Here's the drawing with two shaded views (mm, measured from the low corner). I have some questions. A direction names the side the tool comes from. Round coordinates to 2 decimals unless told otherwise and drop trailing zeros. Loops run counter-clockwise (first coordinate to the right, second up) from the corner with the lowest first, then second, coordinate; pieces in that order, holes last. Notation, with made-up numbers: M 7,37.5 L 65,37.5 A7 cw 65,46.5 Z; hole C 46.5,14 d9. An arc over 180 degrees is marked long. Write each question's results on one line, items separated by ' | '. Start each with the question number.
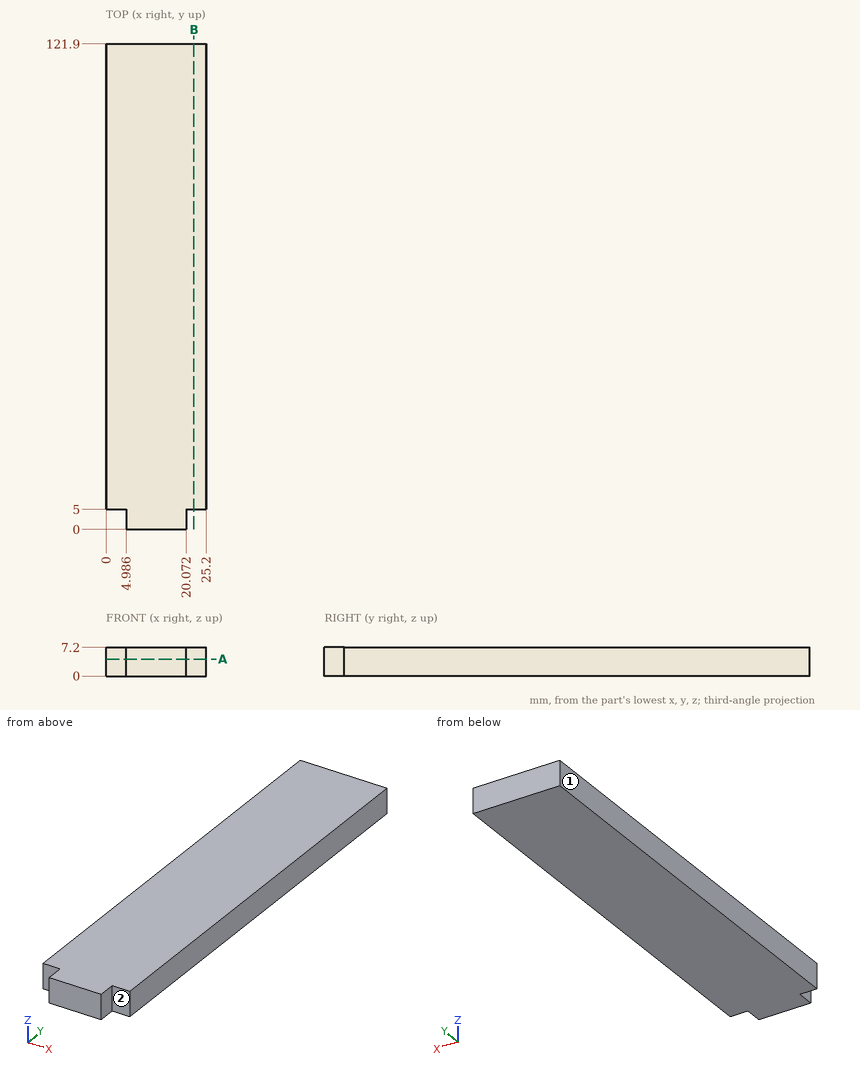
Item 1: Which directions (+Z, -Z, +X, -X, +Y, -Y) give clear straight access to the entire face, cutting with the end or side of a thin tool? Please do the marked faces 1 and 2.
Item 2: If we section it at A-A on z = 4.25: Please give me the cut outline in (x, y), and give its area (3 significant figures).
Item 3: I need wall thicknesses on L1, parallel to Y at x = 20.25, z = 5.75. Which ranges of the line are inside material? Lowest first, please.
Item 4: If we section it at B-B on x = 22: Please give me the cut outline in (y, z).
Item 5: I'm going to push flat-ended pins straight in: pin 1 (4 mm diameter, centred on x = 23, z = 4.5, fed in from -Y); pin 2 (1.5 mm diameter, centred on y = 1.5, z = 3.5, fed in from -X). Where does each tip first touch, or does it pass through?
Numbers:
1) face 1: +Z, -Z, -X, +Y, -Y | face 2: +Z, -Z, +X, -Y
2) outline: M 0,5 L 4.99,5 L 4.99,0 L 20.07,0 L 20.07,5 L 25.2,5 L 25.2,121.9 L 0,121.9 Z | area: 3,020 mm²
3) L1: 5 to 121.9
4) outline: M 5,0 L 121.9,0 L 121.9,7.2 L 5,7.2 Z
5) pin 1: y = 5 | pin 2: x = 4.99
